Verification items for the finished model (mm, model axes). Face numbers are marked on the shaded views. A direction names the side the tool comes from. Coordinates: 2 decimals unless noted, no trailing zeros. Write each loop counter-clockwise with the first axis right and the second up, starting at its lowest first coordinate (ties: lowest second). Pieces come first, ordered by that corner, then holes. Notation, with made-up numbers: M -7,20.25 L 47,20.25 A10 ccw 47,30.25 Z; hole C -39.75,66 d9. An arc over 180 degrees is marked long. Answer in a Markdown table with one row per item.
from build123d import *

# Parameters (mm, degrees)
F0_W     = 2387.6
F0_H     = 1117.6
F1_DEPTH = 670
F3_DEPTH = 711.2
F4_R     = 76.19999
F5_SIZE  = 50.8


# Not quite as in the source:
# - a fillet or chamfer is up to 0.001 mm smaller than in the source, because OpenCascade refuses the exact size


with BuildPart() as f1:
    # F0 (on Top) → F1 (new body)
    with BuildSketch(Plane.XY):
        with Locations((-1193.8, 558.8)):
            Rectangle(F0_W, F0_H)
    extrude(amount=F1_DEPTH)

    # F2 (on face) → F3 (cut)
    with BuildSketch(Plane.XZ):
        Polygon((-2235.2, 300), (-152.4, 300), (-152.4, 485), (0, 485), (0, 670), (-152.4, 670), (-2235.2, 670), (-2387.6, 670), (-2387.6, 485), (-2235.2, 485), align=None)
    extrude(amount=-F3_DEPTH, mode=Mode.SUBTRACT)

    # F4 (radius 76.2 in the source; OpenCascade refuses exactly that, so slightly less here)
    f4_edges = [f1.edges().sort_by_distance(p)[0] for p in [
        (-2235.2, 355.6, 485),
        (-1193.8, 711.2, 670),
        (-152.4, 355.6, 485),
        (0, 355.6, 485),
        (-1193.8, 1117.6, 670),
        (-2387.6, 355.6, 485),
        (-2387.6, 711.2, 577.5),
        (0, 711.2, 577.5),
    ]]
    fillet(f4_edges, radius=F4_R)

    # F5
    f5_edges = [f1.edges().sort_by_distance(p)[0] for p in [
        (-1193.8, 711.2, 300),
        (-2235.2, 355.6, 300),
        (-152.4, 355.6, 300),
        (-1193.8, 0, 300),
        (0, 0, 204.400005),
        (-22.31846, 0, 462.68154),
        (-76.2, 0, 485),
        (-2387.6, 0, 204.400005),
        (-130.08154, 0, 462.68154),
        (-2365.28154, 0, 462.68154),
        (-2311.4, 0, 485),
        (-2257.51846, 0, 462.68154),
    ]]
    chamfer(f5_edges, length=F5_SIZE)


solid = f1.part
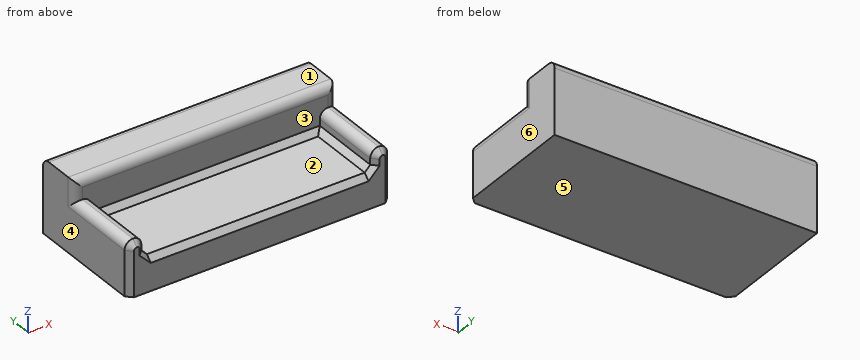
1) Tool access check on the marked faces 1 and 2. Record the directions out of +Z, -Z, +X, -X, +Y, -Y that give a thin tool (end or side, any length) a straight path to the whole face; none if there is none.
Response values:
| item | result |
|---|---|
| face 1 | +Z, +X, -X, +Y, -Y |
| face 2 | +Z, -Y |
2) Sectioned sample at B-B (z = 326). Record the cut outline in (x, y).
Response values:
| item | result |
|---|---|
| outline | M -2387.6,50.8 L -2336.8,0 L -2261.2,0 L -2210.4,50.8 L -2210.4,686.4 L -177.2,686.4 L -177.2,50.8 L -126.4,0 L -50.8,0 L 0,50.8 L 0,1117.6 L -2387.6,1117.6 Z |
3) Release check for a two-part mould opening along X. For the marked faces 3, 4, 5 and 6 record: +X half, -X half, draft (parallel to the pull), parting line (faces both ways), or undercut.
Response values:
| item | result |
|---|---|
| face 3 | undercut |
| face 4 | -X half |
| face 5 | draft |
| face 6 | +X half |
4) Sectioned sample at A-A (x = -1229). Record the cut outline in (y, z).
Response values:
| item | result |
|---|---|
| outline | M 0,0 L 1117.6,0 L 1117.6,593.8 A76.2 ccw 1041.4,670 L 787.4,670 A76.2 ccw 711.2,593.8 L 711.2,350.8 L 660.4,300 L 50.8,300 L 0,249.2 Z |
5) Depth check by flat-ended pin: pin 1 (1.5 mm diameter, centred on x = -1587.5, y = 143, fed in from +Z); pin 2 (3 mm diameter, centred on x = -385, z = 501, fed in from -Y). Enter the tip coordinate at first touch or a pass-through.
Response values:
| item | result |
|---|---|
| pin 1 | stops at z = 300 |
| pin 2 | stops at y = 711.2 |
6) Thickness scan on L1, parallel to X at y = 358, z = 354; L2, parallel to Z at x = -575, y = 218; L3, parallel to Y at x = -1844, z = 414. Record the ranges inside material, lowest first. Write a range as [from, to].
Response values:
| item | result |
|---|---|
| L1 | x = [-2387.6, -2235.2], [-152.4, 0] |
| L2 | z = [0, 300] |
| L3 | y = [711.2, 1117.6] |
7) Sectioned sample at D-D (z = 617). Record the cut outline in (x, y), then the cut area to 3 significant figures.
Response values:
| item | result |
|---|---|
| outline | M -2387.6,787.4 A76.2 ccw -2334.6,714.82 L -53,714.82 A76.2 ccw 0,787.4 L 0,1113.98 L -2387.6,1113.98 Z |
| area | 951,000 mm² |
